The listing builds one solid part. Answer for the finished solid, in the listing's coordinates (mm). Face numbers are marked on the shaded views. A direction names the side the tool comes from. Coordinates: 2 decimals unless noted, no trailing zeros. Loops run counter-clockwise (first coordinate to the right, second up) from the corner with the lowest first, then second, coordinate; pieces in that order, holes last. Notation, with made-up numbers: M 55.5,77 L 107.5,77 A17 ccw 107.5,107 Z; hole C 24.5,66.5 d9. An arc over 180 degrees is marked long. Return JSON: item names as keys, results as strings. Group by question number.
1. The mould has two halves that part along Z. Classify the marked faces 1, 2, 3 and 4: pulls with the +Z half, pulls with the -Z half, needs draft (parallel to the pull), parting line crosses it, or undercut.
2. Straight lines are drawn through the part: L1, parallel to Z at x = 48, y = -7; L2, parallel to X at y = -59.5, z = 8.5; L3, parallel to X at y = -19, z = 16. For each, find the intervals that lie inside material, in ascending order. Write a range as from..to.
3. Section D-D (z = -31.5) is taken. Write down the section's boundary in (x, y), then the cut area to 3 significant figures.
4. Section C-C (y = -39.5) is taken. Write down the section's boundary in (x, z).
5. Section A-A (x = 55) is taken. Write down the section's boundary in (y, z).
6. Section B-B (z = 0) is taken. Write down the section's boundary in (x, y), then the cut area to 3 significant figures.
7. Which of the six approach directions +Z, -Z, +X, -X, +Y, -Y give full straight-line access (tool end or side, diameter ignored) to the marked faces 5 and 6?
8. Given P1, Ø2.5, axis at x = 1.5, z = -46, coming from the +Y side; P2, Ø4, axis at x = -2.5, z = 46.5, coming from the +Y side, each flat-ended and moving along its own axis, determine where each tip first touches the part or whether it passes through.
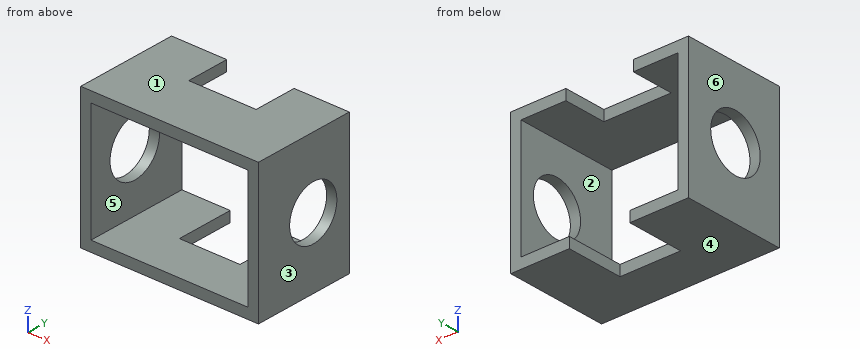
```python
from build123d import *

# Parameters (mm, degrees)
F0_W      = 131.0027092695
F0_H      = 102.4924069643
F1_DEPTH  = 76.2
F2_W      = 115.8900782466
F2_H      = 86.941331625
F3_DEPTH  = 38.1
F4_DEPTH  = 25.4
F5_DEPTH  = 76.2
F6_W      = 44.6236804128
F6_H      = 42.5505377352
F7_DEPTH  = 76.2
F8_W      = 49.6712476015
F8_H      = 31.8642035127
F9_DEPTH  = 76.2
F10_R     = 20.7740472605
F11_DEPTH = 76.2
F12_R     = 19.8125054643
F13_DEPTH = 25.4


with BuildPart() as f1:
    # F0 (on Front) → F1 (new body)
    with BuildSketch(Plane.XZ):
        Rectangle(F0_W, F0_H)
    extrude(amount=F1_DEPTH)

    # F2 (on Front) → F3 (cut, symmetric)
    with BuildSketch(Plane.XZ):
        Rectangle(F2_W, F2_H)
    extrude(amount=F3_DEPTH, both=True, mode=Mode.SUBTRACT)

    # F4 (cut): a face of the model
    f4_faces = [f1.faces().sort_by_distance(p)[0] for p in [
        (0, -38.1, 0),
    ]]
    extrude(f4_faces, amount=-F4_DEPTH, mode=Mode.SUBTRACT)

    # F5 (cut): a face of the model
    f5_faces = [f1.faces().sort_by_distance(p)[0] for p in [
        (0, -63.5, 0),
    ]]
    extrude(f5_faces, amount=-F5_DEPTH, mode=Mode.SUBTRACT)

    # F6 (on Top) → F7 (cut)
    with BuildSketch(Plane.XY):
        with Locations((0, -21.2752688676)):
            Rectangle(F6_W, F6_H)
    extrude(amount=-F7_DEPTH, mode=Mode.SUBTRACT)

    # F8 (on face) → F9 (cut)
    with BuildSketch(Plane.XY.offset(51.2462034822)):
        with Locations((0, -15.9321017563)):
            Rectangle(F8_W, F8_H)
    extrude(amount=-F9_DEPTH, mode=Mode.SUBTRACT)

    # F10 (on Right) → F11 (cut)
    with BuildSketch(Plane.YZ):
        with Locations((-39.45556283, 0)):
            Circle(F10_R)
    extrude(amount=-F11_DEPTH, mode=Mode.SUBTRACT)

    # F12 (on face) → F13 (cut)
    with BuildSketch(Plane.YZ.offset(65.5013546348)):
        with Locations((-30.2042365074, 0)):
            Circle(F12_R)
    extrude(amount=-F13_DEPTH, mode=Mode.SUBTRACT)


solid = f1.part
```
Worked out:
{
 "1": {"face 1": "pulls with the +Z half", "face 2": "undercut", "face 3": "needs draft", "face 4": "pulls with the -Z half"},
 "2": {"L1": "-51.25..-43.47, 43.47..51.25", "L2": "-65.5..-57.95, 57.95..65.5", "L3": "-65.5..-57.95"},
 "3": {"outline": "M -65.5,-76.2 L -57.95,-76.2 L -57.95,0 L -65.5,0 Z; M 57.95,-76.2 L 65.5,-76.2 L 65.5,0 L 57.95,0 Z", "area": "1,150 mm^2"},
 "4": {"outline": "M -65.5,-51.25 L -22.31,-51.25 L -22.31,-43.47 L -57.95,-43.47 L -57.95,-20.77 L -65.5,-20.77 Z; M -65.5,20.77 L -57.95,20.77 L -57.95,43.47 L 57.95,43.47 L 57.95,17.5 L 65.5,17.5 L 65.5,51.25 L -65.5,51.25 Z; M 22.31,-51.25 L 65.5,-51.25 L 65.5,-17.5 L 57.95,-17.5 L 57.95,-43.47 L 22.31,-43.47 Z"},
 "5": {"outline": "M -76.2,-51.25 L 0,-51.25 L 0,-43.47 L -76.2,-43.47 Z; M -76.2,43.47 L 0,43.47 L 0,51.25 L -76.2,51.25 Z"},
 "6": {"outline": "M -65.5,-76.2 L -57.95,-76.2 L -57.95,-60.23 L -65.5,-60.23 Z; M -65.5,-18.68 L -57.95,-18.68 L -57.95,0 L -65.5,0 Z; M 57.95,-76.2 L 65.5,-76.2 L 65.5,-50.02 L 57.95,-50.02 Z; M 57.95,-10.39 L 65.5,-10.39 L 65.5,0 L 57.95,0 Z", "area": "538 mm^2"},
 "7": {"face 5": "+Y, -Y", "face 6": "+Z, -Z, -X, +Y, -Y"},
 "8": {"P1": "y = -42.55", "P2": "y = -31.86"}
}
